Autodesk Inventor part; units mm, degrees
ref_plane "YZ Plane" through (0, 0, 0) normal (1, 0, 0) x (0, 1, 0)
ref_plane "XZ Plane" through (0, 0, 0) normal (0, 1, 0) x (-1, 0, 0)
ref_plane "XY Plane" through (0, 0, 0) normal (0, 0, 1) x (1, 0, 0)
sketch "Sketch1" plane through (0, 0, 0) normal (0, 0, 1) x (1, 0, 0)
  line L0 (22.0635, 29.031) -> (22.0741, 29.031)
  line L1 (22.0635, 29.031) -> (22.0635, 28.8989)
  arc A0 (22.0635, 28.8989) -> (22.0653, 28.8449) centre (22.893, 28.8989) ccw
  line L2 (22.893, 28.0694) -> (48.1914, 28.0694)
  arc A1 (48.6061, 27.6547) -> (48.1914, 28.0694) centre (48.6061, 28.0694) ccw
  line L3 (48.6061, 27.6547) -> (48.6061, 26.4105)
  line L4 (48.6061, 26.4105) -> (42.7999, 26.4105)
  arc A2 (42.7999, 26.4105) -> (41.9705, 25.581) centre (42.7999, 25.581) ccw
  line L5 (41.9705, 25.581) -> (41.9705, 23.4245)
  line L6 (29.5286, 23.4245) -> (41.9705, 23.4245)
  line L7 (29.5286, 25.6909) -> (29.5286, 23.4245)
  line L8 (22.0635, 25.6909) -> (29.5286, 25.6909)
  line L9 (22.0635, 33.3622) -> (52.8128, 33.3622)
  line L10 (52.8128, 33.3622) -> (52.8128, 19.4198)
  line L11 (52.8128, 19.4198) -> (22.0635, 19.4198)
  line L12 (22.0635, 19.4198) -> (22.0635, 33.3622)
  line L13 (21.7606, 28.8449) -> (22.0653, 28.8449)
  line L14 (56.2668, 28.0694) -> (56.2411, 28.0694)
  line L15 (22.0635, 25.6909) -> (30.348, 25.6909)
  line L16 (42.7999, 26.4105) -> (48.6061, 26.4105)
  line L17 (22.0635, 34.9405) -> (22.0635, 17.9582)
  line L18 (17.0806, 21.0245) -> (52.8128, 21.0245)
  line L19 (48.1914, 28.0694) -> (22.0635, 28.0694)
  line L20 (14.2529, 30.3694) -> (52.8128, 30.3694)
  dimension "d0" = 2.4
  dimension "d2" = 2.3
extrude "Extrusion1" add sketch "Sketch1" along normal blind 10 contours L12 L20 L10 L18 L8 L7 L6 L5 A2 L4 L3 A1 L2 L19 A0 L1 | L12 L9 L10 L20 | L10 L11 L12 L18
sketch "Sketch2" plane through (0, 0, 10) normal (0, 0, 1) x (1, 0, 0)
  line L0 (22.0635, 28.0694) -> (48.1914, 28.0694)
  line L1 (41.9705, 23.4245) -> (29.5286, 23.4245)
  line L2 (22.0635, 25.6909) -> (22.0635, 19.4198)
  line L3 (52.8128, 19.4198) -> (52.8128, 33.3622)
  line L4 (22.0635, 33.3622) -> (52.8128, 33.3622)
  line L5 (52.8128, 33.3622) -> (52.8128, 30.5694)
  line L6 (52.8128, 30.5694) -> (22.0635, 30.5694)
  line L7 (22.0635, 30.5694) -> (22.0635, 33.3622)
  line L8 (52.8128, 19.4198) -> (22.0635, 19.4198)
  line L9 (22.0635, 19.4198) -> (22.0635, 21.1245)
  line L10 (22.0635, 21.1245) -> (52.8128, 21.1245)
  line L11 (52.8128, 21.1245) -> (52.8128, 19.4198)
  point P0 (0, 0)
  dimension "d5" = 2.5
  dimension "d6" = 2.3
extrude "Extrusion2" cut sketch "Sketch2" against normal blind 10
fillet "Fillet1" radius 2 3 edges at (52.8128, 30.5694, 5) (52.8128, 21.1245, 5) (22.0635, 21.1245, 5)
sketch "Sketch3" plane through (22.0635, 30.5694, 10) normal (0, 1, 0) x (1, 0, 0)
  line L0 (0, 0) -> (0, 10)
  circle A0 centre (3.2, 5) radius 1.7
  point P0 (-22.0635, 10)
  dimension "d10" = 3.4
  dimension "d11" = 3.2
extrude "Extrusion3" cut sketch "Sketch3" against normal blind 10
sketch "Sketch4" plane through (29.5286, 23.4245, 0) normal (0, 1, 0) x (1, 0, 0)
  line L0 (0, 0) -> (12.4418, 0)
  line L1 (0, 0) -> (0, -10)
  line L2 (12.4418, -10) -> (0, -10)
  line L3 (12.4418, 0) -> (12.4418, -10)
  point P0 (-29.5286, 0)
extrude "Extrusion4" add sketch "Sketch4" along normal blind 1.4
properties part number "Loop"
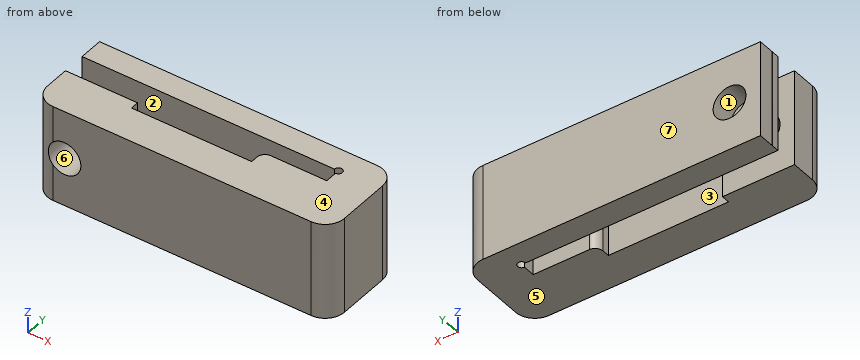
For this review, take the finished solid that the model builds, in its own axes (mm). Face numbers are marked on the shaded views. A direction names the side the tool comes from. Give positions to 0.01 mm unless a question says otherwise; leave off trailing zeros. Order: outer loops, then holes, each group sorted by start corner. A loop starts at its lowest first (then second) coordinate and runs counter-clockwise, first axis right, second up. Notation, with made-up numbers: (61.5, 79.25) -> (111.5, 79.25) arc R25 cw to (111.5, 106.25) -> close; hole circle Ø5 at (-19.75, -33.5). An arc over 180 degrees is marked (long way). Write item = value, one per line.
1) We need section A-A, the plane x = 39. Give the boundary of the cut face in (y, z), and give its area (3 significant figures).
Findings:
outline = (21.12, 0) -> (24.82, 0) -> (24.82, 10) -> (21.12, 10) -> close; (28.07, 0) -> (30.57, 0) -> (30.57, 10) -> (28.07, 10) -> close
area = 62.0 mm^2
2) We need section D-D, the plane x = 25. Give the boundary of the cut face in (y, z), and give its area (3 significant figures).
Findings:
outline = (21.12, 0) -> (25.69, 0) -> (25.69, 3.32) -> (21.12, 3.32) -> close; (21.12, 6.68) -> (25.69, 6.68) -> (25.69, 10) -> (21.12, 10) -> close; (28.07, 0) -> (30.57, 0) -> (30.57, 3.32) -> (28.07, 3.32) -> close; (28.07, 6.68) -> (30.57, 6.68) -> (30.57, 10) -> (28.07, 10) -> close
area = 46.9 mm^2
3) Insertion check: pin 1 (3 mm diameter, centred on x = 25.26, z = 5, fed in from -Y). The pin has a flat end and moves straight along its axis. Give the tip position at first contact, or say it passes through.
Findings:
pin_1 = through
4) We need section B-B, the plane z = 4.5. Give the boundary of the cut face in (x, y), and give its area (3 significant figures).
Findings:
outline = (22.06, 23.12) arc R2 ccw to (23.64, 21.17) -> (23.64, 25.69) -> (22.06, 25.69) -> close; (22.06, 28.07) -> (23.64, 28.07) -> (23.64, 30.57) -> (22.06, 30.57) -> (22.06, 28.9) arc R0.79 ccw to (22.07, 28.84) -> close; (26.89, 21.12) -> (50.81, 21.12) arc R2 ccw to (52.81, 23.12) -> (52.81, 28.57) arc R2 ccw to (50.81, 30.57) -> (26.89, 30.57) -> (26.89, 28.07) -> (48.19, 28.07) arc R0.41 cw (long way) to (48.61, 27.65) -> (48.61, 26.41) -> (42.8, 26.41) arc R0.83 ccw to (41.97, 25.58) -> (41.97, 24.82) -> (29.53, 24.82) -> (29.53, 25.69) -> (26.89, 25.69) -> close
area = 195 mm^2
5) To check wall thickness, follow L1, parallel to Y at x = 41, z = 7; L2, parallel to Y at x = 28.5, z = 8.75; L3, parallel to X at y = 25, z = 5.75. State the ranges of each line that lie inside material, in increasing order. Write a range as from..to.
Findings:
L1 = 21.12..24.82, 28.07..30.57
L2 = 21.12..25.69, 28.07..30.57
L3 = 22.06..23.74, 26.79..29.53, 41.97..52.81
6) We need section C-C, the plane y = 24. Give the boundary of the cut face in (x, z), and give its area (3 significant figures).
Findings:
outline = (22.06, 0) -> (52.81, 0) -> (52.81, 10) -> (22.06, 10) -> close; hole circle Ø3.4 at (25.26, 5)
area = 298 mm^2
7) For the marked faces 1, 2 and 3, list the 3-axis set-ups (+Z, -Z, +X, -X, +Y, -Y) from which the entire face can be reached by the end or side of a thin tool; tool diameter is ignored.
Findings:
face_1 = +Y, -Y
face_2 = +Z, -Z, -X
face_3 = +Z, -Z
8) Draft analysis for pull direction Z (two halves, no side actions). For the marked faces 4, 5, 6 and 7, state which applies: pulls with the +Z half, pulls with the -Z half, needs draft (parallel to the pull), parting line crosses it, or undercut.
Findings:
face_4 = pulls with the +Z half
face_5 = pulls with the -Z half
face_6 = undercut
face_7 = needs draft
